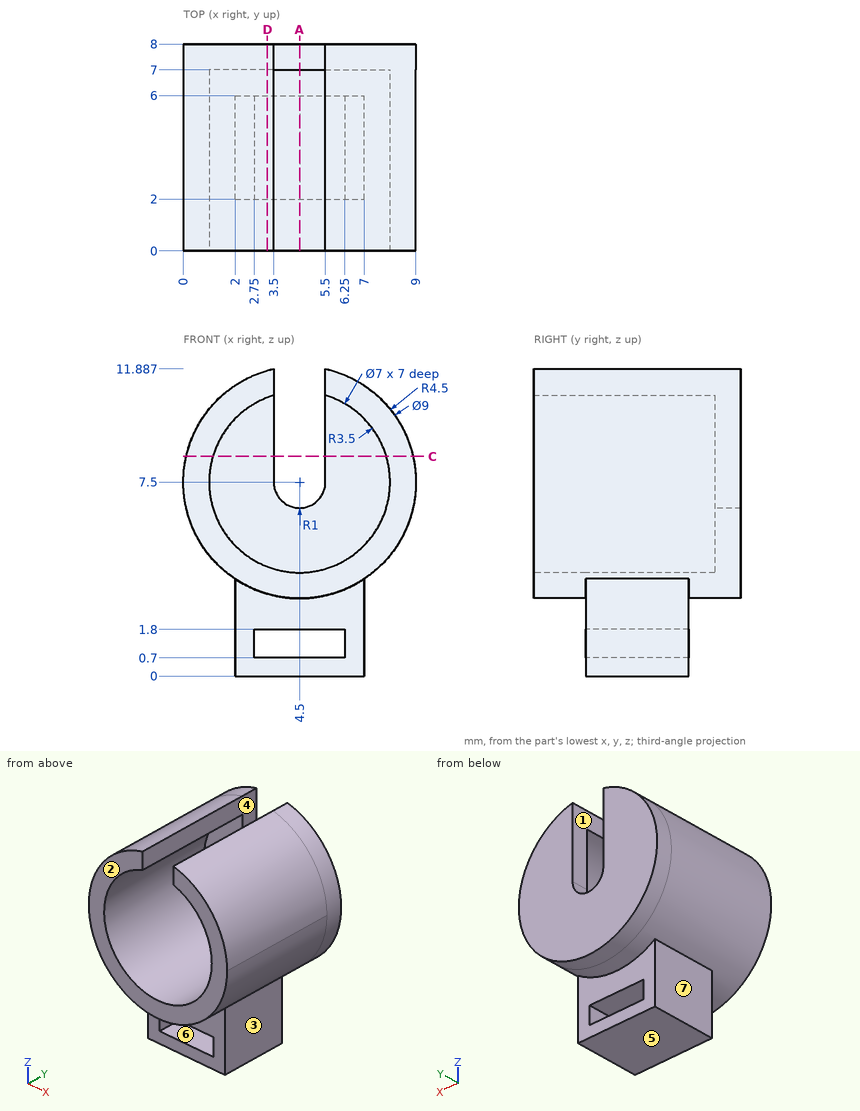
Geometry check sheet. Reference: drawing and pictorial views, mm from the part's lowest x, y, z. A direction names the side the tool comes from. Round coordinates to 2 decimals unless told otherwise and drop trailing zeros. Write each loop counter-clockwise with the first axis right and the second up, starting at its lowest first coordinate (ties: lowest second). Pieces come first, ordered by that corner, then holes.
1. Section check C-C on z = 8.5. Enter the section's corners in (x, y) (1 decimal).
2. Scan lines: L1, parallel to X at y = 5.25, z = 7.5; L2, parallel to Y at x = 7.75, z = 6.5; L3, parallel to X at y = 2.75, z = 11. Record each from-to range of solid material in increasing order.
3. Draft check along X on the marked faces 1, 2, 3 and 4. Enter one of: +X half, -X half, draft (parallel to the pull), parting line (faces both ways), or undercut.
4. Section check A-A on x = 4.5. Enter the section's corners in (y, z), plus the area to 3 significant figures.
5. Section check D-D on x = 3.25. Enter the section's corners in (y, z).
6. Gauge pin test, flat ends, axial feed: P1, Ø4, axis at x = 3.5, z = 1, coming from the -Y side; P2, Ø1, axis at x = 6.5, y = 6, coming from the +Z side; P3, Ø3, axis at x = 6.5, y = 5, coming from the +Z side. Record the tip position at first contact, or that the pin passes through.
7. Access from +Z, -Z, +X, -X, +Y, -Y to the whole of each face (thin tool, end or side, straight path). Record for the marked faces 5, 6 and 7.
Answer:
1. outline: (0.1, 0) - (1.1, 0) - (1.1, 7) - (3.5, 7) - (3.5, 8) - (0.1, 8) - close; (5.5, 7) - (7.9, 7) - (7.9, 0) - (8.9, 0) - (8.9, 8) - (5.5, 8) - close
2. L1: x = 0 to 1, 8 to 9
2. L2: y = 7 to 8
2. L3: x = 1.67 to 3.5, 5.5 to 7.33
3. face 1: undercut
3. face 2: draft
3. face 3: +X half
3. face 4: undercut
4. outline: (0, 3) - (2, 3) - (2, 1.8) - (6, 1.8) - (6, 3) - (8, 3) - (8, 6.5) - (7, 6.5) - (7, 4) - (0, 4) - close; (2, 0) - (6, 0) - (6, 0.7) - (2, 0.7) - close
4. area: 18.1 mm2
5. outline: (0, 3.18) - (2, 3.18) - (2, 1.8) - (6, 1.8) - (6, 3.18) - (8, 3.18) - (8, 11.82) - (0, 11.82) - (0, 10.77) - (7, 10.77) - (7, 4.23) - (0, 4.23) - close; (2, 0) - (6, 0) - (6, 0.7) - (2, 0.7) - close
6. P1: stops at y = 2
6. P2: stops at z = 11.74
6. P3: stops at z = 11.89
7. face 5: -Z, +X, -X, +Y, -Y
7. face 6: +Y, -Y
7. face 7: -Z, -X, +Y, -Y
